Source: CAD feature listing. Evaluate the final solid. Frame: model axes, mm. Face numbers are marked on the shaded views. A direction names the side the tool comes from. Give positions to 0.01 mm unless a question says otherwise; leave off trailing zeros. Write each loop counter-clockwise with the first axis right and the second up, starting at its lowest first coordinate (ties: lowest second). Pieces come first, ordered by that corner, then holes. Notation, with made-up numbers: (14.25, 33) - (70.25, 33) arc R20 cw to (70.25, 67) - close; hole circle Ø11 at (57, -2). An arc over 180 degrees is marked (long way). One line per question, with ' | ' between items. Start each with the question number.
(1) Ray query, line 1 (Z direction, x = -118, y = 24.35); line 2 (X direction, y = -11, z = -5); line 3 (Z direction, x = -124.3, y = -15.5). Return the intervals inside material, ascending. Write a range as [from, to].
(2) Section C-C, the plane z = 15.5. Return loops of the section in (x, y), plus the area to 3 significant figures.
(3) Access query for the marked faces 1 and 2. Directions: +Z, -Z, +X, -X, +Y, -Y. A direction counts if a zero-diameter tool reaches every point of the face in a straight line with its end or side. Return the directions, or none.
(4) Draft query along X for the marked faces 3, 4 and 5. Return one class per face: +X half, -X half, draft (parallel to the pull), parting line (faces both ways), or undercut.
(5) Pin query (flat end, axial travel): pin 1 (5 mm diameter, centred on x = -4, z = -22, fed in from +Y); pin 2 (2 mm diameter, centred on x = 2, y = 4.5, fed in from +Z). Return the tip coordinate at first contact, or that it passes through.
(6) Section B-B, the plane x = -114. Return loops of the section in (y, z), plus the area to 3 significant figures.
(7) Section D-D, the plane y = -18.5. Return loops of the section in (x, z), plus the area to 3 significant figures.
(8) Section A-A, the plane y = 0. Return loops of the section in (x, z).
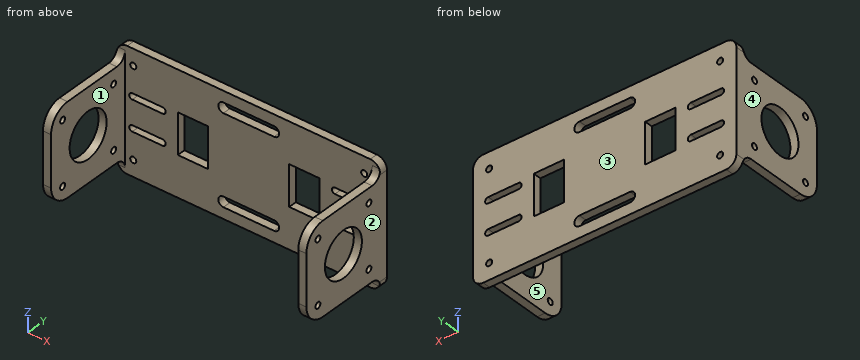
Autodesk Inventor part; units mm, degrees
ref_plane "Mid Plane" through (-61, 26.5, 30) normal (-1, 0, 0) x (0, 0, 1)
ref_plane "YZ Plane" through (0, 0, 0) normal (1, 0, 0) x (0, 1, 0)
ref_plane "XZ Plane" through (0, 0, 0) normal (0, 1, 0) x (-1, 0, 0)
sketch "Motor Support" plane through (0, 0, 0) normal (1, 0, 0) x (0, 1, 0)
  circle A0 centre (0, 0) radius 11.25
  line L0 (-12.5, -22.5) -> (22.5, -22.5)
  line L1 (22.5, -22.5) -> (22.5, 22.5)
  line L2 (22.5, 22.5) -> (-12.5, 22.5)
  line L3 (-22.5, 12.5) -> (-22.5, -12.5)
  arc A1 (-12.5, 22.5) -> (-22.5, 12.5) centre (-12.5, 12.5) ccw
  arc A2 (-22.5, -12.5) -> (-12.5, -22.5) centre (-12.5, -12.5) ccw
  circle A3 centre (15.5, 15.5) radius 1.5
  circle A4 centre (15.5, -15.5) radius 1.5
  circle A5 centre (-15.5, 15.5) radius 1.5
  circle A6 centre (-15.5, -15.5) radius 1.5
  point P0 (-22.5, 22.5)
  point P1 (22.5, 0)
  dimension "d0" = 22.5
  dimension "d1" = 45
  dimension "d2" = 45
  dimension "d3" = 10
  dimension "d4" = 22.5
  dimension "d5" = 3
  dimension "d6" = 3
  dimension "d7" = 3
  dimension "d8" = 3
  dimension "d9" = 31
  dimension "d10" = 31
  dimension "d11" = 15.5
  dimension "d12" = 15.5
extrude "Motor Support E" add sketch "Motor Support" along normal blind 4
sketch "Base" plane through (0, 22.5, 22.5) normal (0, 1, 0) x (1, 0, 0)
  line L0 (0, 45) -> (0, 0)
  line L1 (0, 0) -> (4, 0)
  line L2 (4, 45) -> (4, 0)
  line L3 (0, 45) -> (4, 45)
  line L4 (4, -7.5) -> (-61, -7.5)
  line L5 (-61, -7.5) -> (-61, 52.5)
  line L6 (-61, 52.5) -> (4, 52.5)
  line L7 (4, 52.5) -> (4, -7.5)
  line L8 (-41, 32.5) -> (-26, 32.5)
  line L9 (-26, 32.5) -> (-26, 12.5)
  line L10 (-26, 12.5) -> (-41, 12.5)
  line L11 (-41, 12.5) -> (-41, 32.5)
  point P0 (0, 22.5)
  point P1 (4, 22.5)
  point P2 (-26, 22.5)
  point P3 (0, 22.5)
  dimension "d15" = 65
  dimension "d16" = 60
  dimension "d19" = 15
  dimension "d20" = 20
  dimension "d21" = 26
extrude "Base E" add sketch "Base" along normal blind 4
ref_plane "Mid Plane" through (-61, 26.5, 30) normal (-1, 0, 0) x (0, 0, 1)
mirror "Mirror Base" about plane through (-61, 26.5, 30) normal (-1, 0, 0)
fillet "Fillet1" radius 5 4 edges at (4, 24.5, 30) (4, 24.5, -30) (-126, 24.5, 30) (-126, 24.5, -30)
fillet "Fillet2" radius 5 4 edges at (2, 22.5, -22.5) (2, 22.5, 22.5) (-124, 22.5, -22.5) (-124, 22.5, 22.5)
sketch "Base Hole Pattern" plane through (0, 26.5, 22.5) normal (0, 1, 0) x (1, 0, 0)
  circle A0 centre (-4, 0.5) radius 1.5
  circle A1 centre (-118, 44.5) radius 1.5
  circle A2 centre (-118, 0.5) radius 1.5
  circle A3 centre (-4, 44.5) radius 1.5
  arc A4 (-121, 52.5) -> (-126, 47.5) centre (-121, 47.5) ccw
  line L0 (-126, -2.5) -> (-126, 47.5)
  arc A5 (-126, -2.5) -> (-121, -7.5) centre (-121, -2.5) ccw
  line L1 (-1, -7.5) -> (-121, -7.5)
  arc A6 (-1, -7.5) -> (4, -2.5) centre (-1, -2.5) ccw
  line L2 (4, -2.5) -> (4, 47.5)
  arc A7 (4, 47.5) -> (-1, 52.5) centre (-1, 47.5) ccw
  line L3 (-1, 52.5) -> (-121, 52.5)
  line L4 (-81, 32.5) -> (-96, 32.5)
  line L5 (-81, 12.5) -> (-81, 32.5)
  line L6 (-96, 12.5) -> (-81, 12.5)
  line L7 (-96, 32.5) -> (-96, 12.5)
  line L8 (-41, 32.5) -> (-26, 32.5)
  line L9 (-26, 32.5) -> (-26, 12.5)
  line L10 (-26, 12.5) -> (-41, 12.5)
  line L11 (-41, 12.5) -> (-41, 32.5)
  line L12 (-73.5, 44.5) -> (-48.5, 44.5) construction
  line L13 (-73.5, 42) -> (-48.5, 42)
  line L14 (-48.5, 47) -> (-73.5, 47)
  arc A8 (-73.5, 47) -> (-73.5, 42) centre (-73.5, 44.5) ccw
  arc A9 (-48.5, 42) -> (-48.5, 47) centre (-48.5, 44.5) ccw
  line L15 (-73.5, 0.5) -> (-48.5, 0.5) construction
  line L16 (-73.5, -2) -> (-48.5, -2)
  line L17 (-48.5, 3) -> (-73.5, 3)
  arc A10 (-73.5, 3) -> (-73.5, -2) centre (-73.5, 0.5) ccw
  arc A11 (-48.5, -2) -> (-48.5, 3) centre (-48.5, 0.5) ccw
  line L18 (-118.5, 30) -> (-103.5, 30) construction
  line L19 (-118.5, 28.5) -> (-103.5, 28.5)
  line L20 (-103.5, 31.5) -> (-118.5, 31.5)
  arc A12 (-118.5, 31.5) -> (-118.5, 28.5) centre (-118.5, 30) ccw
  arc A13 (-103.5, 28.5) -> (-103.5, 31.5) centre (-103.5, 30) ccw
  line L21 (-118.5, 15) -> (-103.5, 15) construction
  line L22 (-118.5, 13.5) -> (-103.5, 13.5)
  line L23 (-103.5, 16.5) -> (-118.5, 16.5)
  arc A14 (-118.5, 16.5) -> (-118.5, 13.5) centre (-118.5, 15) ccw
  arc A15 (-103.5, 13.5) -> (-103.5, 16.5) centre (-103.5, 15) ccw
  line L24 (-18.5, 30) -> (-3.5, 30) construction
  line L25 (-18.5, 28.5) -> (-3.5, 28.5)
  line L26 (-3.5, 31.5) -> (-18.5, 31.5)
  arc A16 (-18.5, 31.5) -> (-18.5, 28.5) centre (-18.5, 30) ccw
  arc A17 (-3.5, 28.5) -> (-3.5, 31.5) centre (-3.5, 30) ccw
  line L27 (-18.5, 15) -> (-3.5, 15) construction
  line L28 (-18.5, 13.5) -> (-3.5, 13.5)
  line L29 (-3.5, 16.5) -> (-18.5, 16.5)
  arc A18 (-18.5, 16.5) -> (-18.5, 13.5) centre (-18.5, 15) ccw
  arc A19 (-3.5, 13.5) -> (-3.5, 16.5) centre (-3.5, 15) ccw
  point P0 (-61, 44.5)
  point P1 (-61, 52.5)
  point P2 (-61, 0.5)
  point P3 (-111, 30)
  point P4 (-111, 15)
  point P5 (-11, 30)
  point P6 (-11, 15)
  dimension "d29" = 3
  dimension "d30" = 3
  dimension "d33" = 3
  dimension "d34" = 3
  dimension "d35" = 8
  dimension "d36" = 8
  dimension "d37" = 8
  dimension "d38" = 8
  dimension "d43" = 25
  dimension "d44" = 5
  dimension "d45" = 25
  dimension "d46" = 2.5
  dimension "d47" = 15
  dimension "d48" = 3
  dimension "d49" = 15
  dimension "d50" = 3
  dimension "d51" = 15
  dimension "d52" = 15
  dimension "d53" = 22.5
  dimension "d56" = 15
  dimension "d57" = 3
  dimension "d58" = 15
  dimension "d59" = 3
  dimension "d60" = 15
  dimension "d61" = 22.5
  dimension "d62" = 15
extrude "Spacer Holes" cut sketch "Base Hole Pattern" against normal blind 10 contours A0 | A1 | A2 | A3
extrude "Base Slots" cut sketch "Base Hole Pattern" against normal blind 10 contours A8 L14 A9 L13 | A10 L17 A11 L16 | A12 L20 A13 L19 | A14 L23 A15 L22 | A16 L26 A17 L25 | A18 L29 A19 L28
equation "\"d6\" = d5"
equation "\"d7\" = d5"
equation "\"d8\" = d5"
equation "\"d30\" = d29"
equation "\"d33\" = d29"
equation "\"d34\" = d29"
equation "\"d36\" = d35"
equation "\"d37\" = d35"
equation "\"d38\" = d35"
equation "\"d45\" = d43"
equation "\"d46\" = 0.5 * d44"
equation "\"d49\" = d47"
equation "\"d50\" = d48"
equation "\"d56\" = d47"
equation "\"d57\" = d48"
equation "\"d58\" = d47"
equation "\"d59\" = d48"
properties part number "Base"
Check sheet entries:
1) line 1: [-30, -23.5], [-20.5, -9], [-6, 6], [9, 20.5], [23.5, 30] | line 2: [-126, -122], [0, 4] | line 3: [-22.04, -17], [-14, 14], [17, 22.04]
2) outline: (-126, -22.04) - (-122, -22.04) - (-122, -17) - (-126, -17) - close; (-126, -14) - (-122, -14) - (-122, 14) - (-126, 14) - close; (-126, 17) - (-122, 17) - (-122, 22.5) - (0, 22.5) - (0, 17) - (4, 17) - (4, 26.5) - (-126, 26.5) - close; (0, -22.04) - (4, -22.04) - (4, -17) - (0, -17) - close; (0, -14) - (4, -14) - (4, 14) - (0, 14) - close | area: 828 mm²
3) face 1: +Z, -Z, -Y | face 2: +Z, -Z, +X, +Y, -Y
4) face 3: draft | face 4: -X half | face 5: undercut
5) pin 1: y = 26.5 | pin 2: z = 22.5
6) outline: (22.5, -30) - (26.5, -30) - (26.5, -9) - (22.5, -9) - close; (22.5, -6) - (26.5, -6) - (26.5, 6) - (22.5, 6) - close; (22.5, 9) - (26.5, 9) - (26.5, 30) - (22.5, 30) - close | area: 216 mm²
7) outline: (-126, -20.5) - (-122, -20.5) - (-122, 20.5) - (-126, 20.5) - close; (0, -20.5) - (4, -20.5) - (4, 20.5) - (0, 20.5) - close | area: 328 mm²
8) outline: (-126, -22.5) - (-122, -22.5) - (-122, -11.25) - (-126, -11.25) - close; (-126, 11.25) - (-122, 11.25) - (-122, 22.5) - (-126, 22.5) - close; (0, -22.5) - (4, -22.5) - (4, -11.25) - (0, -11.25) - close; (0, 11.25) - (4, 11.25) - (4, 22.5) - (0, 22.5) - close
